Geometry: final body of the model. Coordinates: model frame, mm. Face numbers are marked on the shaded views. Round coordinates to 2 decimals unless told otherwise and drop trailing zeros. Order: outer loops, then holes, each group sorted by start corner. A loop starts at its lowest first (then second) coordinate and runs counter-clockwise, first axis right, second up. Notation, with made-up numbers: M 70,-31.5 L 74,-31.5 A15 ccw 74,-5.5 Z; hole C 58.5,35 d9. An arc over 180 degrees is marked long. Put each result on its own line as item: value. Start each with the question number.
1) Section B-B, the plane x = -167. Return loops of the section in (y, z).
2) First-contact query: P1, Ø6, axis at x = -99, z = -69.5, coming from the +Y side; P2, Ø4, axis at x = -130, z = -129, coming from the +Y side; P3, Ø4, axis at y = 25, z = -41.5, coming from the -X side; P4, Ø12, axis at y = 58.5, z = 28, coming from the +X side. Flat tips, straight axial feed; report the tip coordinate or a pass-through.
3) Section D-D, the plane y = 26.5. Return loops of the section in (x, z) (3 decimals), then the cut area to 3 significant figures.
4) Draft query along Z for the marked faces 1, 2, 3 and 4. Return one class per face: pulls with the +Z half, pulls with the -Z half, needs draft (parallel to the pull), parting line crosses it, or undercut.
5) Section C-C, the plane z = -68. Return loops of the section in (x, y).
6) Section A-A, the plane z = 46.5. Return loops of the section in (x, y), then the cut area to 3 significant figures.
7) Material intervals for probe 1 along Y at (x, z) = (-66.5, -135); probe 2 along Z at (x, y) = (-159, 16); probe 3 along Z at (x, y) = (-153.5, 12), sorted ascending. Write a range as [from, to].
from build123d import *

# Parameters (mm, degrees)
BOSS_EXTRUDE3_DEPTH = 3
BOSS_EXTRUDE4_DEPTH = 70
SKETCH6_R           = 5
CUT_EXTRUDE2_DEPTH  = 10


with BuildPart() as part:
    # Sketch1 → Boss-Extrude3 (new body)
    with BuildSketch(Plane(origin=(0, 0, 0), x_dir=(1, 0, 0), z_dir=(0, 1, 0))):
        with BuildLine():
            Line((0, 105), (0, 181))
            ThreePointArc((0, 181), (-167.222195385, 69.265701258), (-127.986327395, -127.986327395))
            Line((-127.986327395, -127.986327395), (-74.246212025, -74.246212025))
            ThreePointArc((-74.246212025, -74.246212025), (-97.007350914, 40.181760398), (0, 105))
        make_face()
    extrude(amount=BOSS_EXTRUDE3_DEPTH)

    # Sketch5 → Boss-Extrude4 (add)
    with BuildSketch(Plane(origin=(0, 3, 0), x_dir=(1, 0, 0), z_dir=(0, 1, 0))):
        with BuildLine():
            Line((0, 181), (0, 178))
            ThreePointArc((0, 178), (-164.450556787, 68.117650961), (-125.865007051, -125.865007051))
            Line((-125.865007051, -125.865007051), (-127.986327395, -127.986327395))
            ThreePointArc((-127.986327395, -127.986327395), (-167.222195385, 69.265701258), (0, 181))
        make_face()
    extrude(amount=BOSS_EXTRUDE4_DEPTH)

    # Sketch6 → Cut-Extrude2 (cut)
    with BuildSketch(Plane(origin=(0, 3, 0), x_dir=(1, 0, 0), z_dir=(0, 1, 0))):
        with Locations((-139.864087078, 6.106597921)):
            Circle(SKETCH6_R)
        with Locations((-111.067352179, -85.224976811)):
            Circle(SKETCH6_R)
        with Locations((-103.216861218, 94.580827618)):
            Circle(SKETCH6_R)
        with Locations((-18.273318865, 138.799636924)):
            Circle(SKETCH6_R)
    extrude(amount=-CUT_EXTRUDE2_DEPTH, mode=Mode.SUBTRACT)


solid = part.part
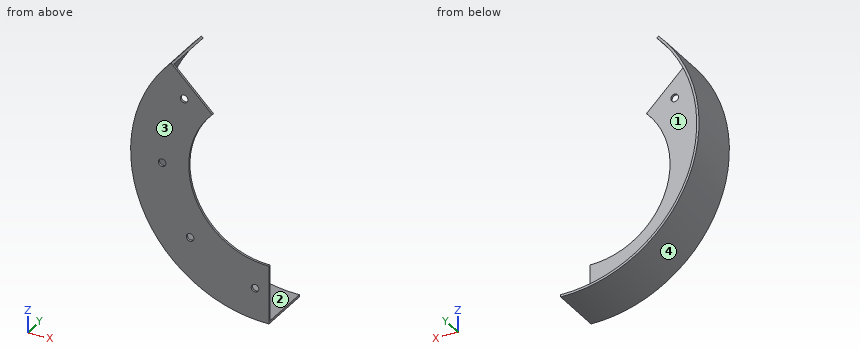
Result sheet:
1. outline: M 0,-69.8 L 73,-69.8 L 73,-61.6 L 3,-61.6 L 3,61.6 L 73,61.6 L 73,69.8 L 0,69.8 Z
2. P1: stops at y = 3
2. P2: passes through
2. P3: stops at x = -176.64
2. P4: stops at x = -174.72
3. outline: M -127.986,127.986 A181 ccw 0,-181 L 0,-178 A178 cw -125.865,125.865 Z
3. area: 1,270 mm2
4. face 1: undercut
4. face 2: undercut
4. face 3: needs draft
4. face 4: parting line crosses it
5. outline: M -167.74,0 L -80.01,0 L -80.01,3 L -164.5,3 L -164.5,73 L -167.74,73 Z
6. outline: M -174.92,0 L -94.14,0 L -94.14,3 L -171.82,3 L -171.82,73 L -174.92,73 Z
6. area: 460 mm2
7. probe 1: y = [0, 3]
7. probe 2: z = [-86.49, -80.02], [80.02, 86.49]
7. probe 3: z = [-95.91, -90.12], [90.12, 95.91]
